Autodesk Inventor part; units mm, degrees
ref_plane "YZ Plane" through (0, 0, 0) normal (1, 0, 0) x (0, 1, 0)
ref_plane "XY Plane" through (0, 0, 0) normal (0, 0, 1) x (1, 0, 0)
sketch "bASE" plane through (0, 0, 0) normal (0, 0, 1) x (1, 0, 0)
  arc A0 (-16.7865, 2.679) -> (-16.7865, -2.679) centre (-16.45, 0) ccw
  arc A1 (16.7865, -2.679) -> (16.7865, 2.679) centre (16.45, 0) ccw
  line L0 (4.4678, -4.2262) -> (16.7865, -2.679)
  line L1 (4.4678, 4.2262) -> (16.7865, 2.679)
  line L2 (-4.4678, 4.2262) -> (-16.7865, 2.679)
  line L3 (-4.4678, -4.2262) -> (-16.7865, -2.679)
  arc A2 (-4.4678, -4.2262) -> (4.4678, -4.2262) centre (0, 0) ccw
  arc A3 (4.4678, 4.2262) -> (-4.4678, 4.2262) centre (0, 0) ccw
  point P0 (0, 4.2262)
  dimension "d20" = 5.4
  dimension "d21" = 5.4
sketch "Coupling" plane through (0, 0, 0) normal (0, 0, 1) x (1, 0, 0)
  line L0 (-4.4678, 4.2262) -> (-16.7865, 2.679)
  arc A0 (4.4678, 4.2262) -> (-4.4678, 4.2262) centre (0, 0) ccw
  line L1 (4.4678, 4.2262) -> (16.7865, 2.679)
  arc A1 (16.7865, -2.679) -> (16.7865, 2.679) centre (16.45, 0) ccw
  line L2 (4.4678, -4.2262) -> (16.7865, -2.679)
  arc A2 (-4.4678, -4.2262) -> (4.4678, -4.2262) centre (0, 0) ccw
  line L3 (-4.4678, -4.2262) -> (-16.7865, -2.679)
  arc A3 (-16.7865, 2.679) -> (-16.7865, -2.679) centre (-16.45, 0) ccw
  line L4 (17.1339, 5.4452) -> (5.7046, 6.8807)
  arc A4 (5.7046, 6.8807) -> (-5.7046, 6.8807) centre (0, 0) ccw
  line L5 (-5.7046, 6.8807) -> (-17.1339, 5.4452)
  arc A5 (-17.1339, 5.4452) -> (-17.1339, -5.4452) centre (-16.45, 0) ccw
  line L6 (-17.1339, -5.4452) -> (-5.7046, -6.8807)
  arc A6 (-5.7046, -6.8807) -> (5.7046, -6.8807) centre (0, 0) ccw
  line L7 (5.7046, -6.8807) -> (17.1339, -5.4452)
  arc A7 (17.1339, -5.4452) -> (17.1339, 5.4452) centre (16.45, 0) ccw
extrude "Extrusion7" add sketch "Coupling" along normal blind 5.5 contours A0 L1 A1 L2 A2 L3 A3 L0 | A7 L7 A6 L6 A5 L5 A4 L4
extrude "Extrusion8" cut sketch "bASE" along normal blind 3
sketch "Sketch8" plane through (0, 0, 3) normal (0, 0, -1) x (-1, 0, 0)
  arc A0 (-4.4678, -4.2262) -> (4.4678, -4.2262) centre (0, 0) ccw
  circle A1 centre (0, 0) radius 4.45
  dimension "d26" = 8.9
extrude "Extrusion9" cut sketch "Sketch8" against normal blind 3
ref_plane "ConstraintPlane" through (0, 0, 0) normal (0, 1, 0) x (-1, 0, 0)
properties part number "ServoHornPocket"
Design review of the part built by this model. Coordinates are the model's own, in mm. A direction names the side the tool comes from. Round coordinates to 2 decimals unless told otherwise and drop trailing zeros. Write each loop counter-clockwise with the first axis right and the second up, starting at its lowest first coordinate (ties: lowest second). Pieces come first, ordered by that corner, then holes. Notation, with made-up numbers: (46, 30) -> (59, 30) arc R32 ccw to (59, 67) -> close; hole circle Ø7 at (-10.75, 45.5). An arc over 180 degrees is marked (long way). One line per item, written item: value. Start each with the question number.
Q1. Add section B-B (y = 0). Give the boundary of the cut face in (x, z), then the cut area to 3 significant figures.
Q2. The part is to be moulded in two halves that separate along X. For faces 1 (the face through (-10.541, 3.463, 1.479)), 2 (the face through (21.937, 0.111, 2.712)), 3 (the face through (-21.937, -0.111, 2.712)), say which applies: pulls with the +X half, pulls with the -X half, needs draft (parallel to the pull), parting line crosses it, or undercut.
Q3. Add section C-C (z = 2.3). Give the boundary of the cut face in (x, y).
Q4. To check wall thickness, follow probe 1 along Y at (x, z) = (0, 5.05); probe 2 along X at (y, z) = (1.75, 3.25); probe 3 along X at (y, z) = (3.75, 3.7). State the ranges of each line that lie inside material, in increasing order.
Q5. Add section D-D (x = 13). Give the boundary of the cut face in (y, z), then the cut area to 3 significant figures.
Q6. Tool access review of faces 4 (the face through (0.087, -8.938, 2.712)), 5 (the face through (0.07, -6.15, 1.48)): name each direction out of +Z, -Z, +X, -X, +Y, -Y from which nothing blocks a thin tool from reaching the whole face with its end or side.
Q7. Add section A-A (x = 0). Give the boundary of the cut face in (y, z), then the cut area to 3 significant figures.
Q8. Insertion check: P1, Ø1, axis at x = 4, z = 4, coming from the +Y side; P2, Ø1.5, axis at x = 13.5, z = 3.5, coming from the -Y side. Each pin has a flat end and moves straight along its axis. Give the tip position at first contact, or say it passes through.
Response:
1. outline: (-21.94, 0) -> (-19.15, 0) -> (-19.15, 3) -> (-4.45, 3) -> (-4.45, 5.5) -> (-21.94, 5.5) -> close; (4.45, 3) -> (19.15, 3) -> (19.15, 0) -> (21.94, 0) -> (21.94, 5.5) -> (4.45, 5.5) -> close
1. area: 104 mm^2
2. face 1: undercut
2. face 2: pulls with the +X half
2. face 3: pulls with the -X half
3. outline: (-17.13, -5.45) -> (-5.7, -6.88) arc R8.94 ccw to (5.7, -6.88) -> (17.13, -5.45) arc R5.49 ccw to (17.13, 5.45) -> (5.7, 6.88) arc R8.94 ccw to (-5.7, 6.88) -> (-17.13, 5.45) arc R5.49 ccw to start; hole (-16.79, -2.68) -> (-4.47, -4.23) arc R6.15 ccw to (4.47, -4.23) -> (16.79, -2.68) arc R2.7 ccw to (16.79, 2.68) -> (4.47, 4.23) arc R6.15 ccw to (-4.47, 4.23) -> (-16.79, 2.68) arc R2.7 ccw to start
4. probe 1: y = -8.94 to -4.45, 4.45 to 8.94
4. probe 2: x = -21.65 to -4.09, 4.09 to 21.65
4. probe 3: x = -20.46 to -2.4, 2.4 to 20.46
5. outline: (-5.96, 0) -> (-3.15, 0) -> (-3.15, 3) -> (3.15, 3) -> (3.15, 0) -> (5.96, 0) -> (5.96, 5.5) -> (-5.96, 5.5) -> close
5. area: 46.7 mm^2
6. face 4: +Z, -Z, -Y
6. face 5: -Z
7. outline: (-8.94, 0) -> (-6.15, 0) -> (-6.15, 3) -> (-4.45, 3) -> (-4.45, 5.5) -> (-8.94, 5.5) -> close; (4.45, 3) -> (6.15, 3) -> (6.15, 0) -> (8.94, 0) -> (8.94, 5.5) -> (4.45, 5.5) -> close
7. area: 39.2 mm^2
8. P1: stops at y = 8.22
8. P2: stops at y = -6
